from build123d import *

# Parameters (mm, degrees)
SKETCH_1_R               = 1.55
SKETCH_1_R_2             = 1.1
EXTRUDE_1_DEPTH          = 3
EXTRUDE_START            = 4.5
SKETCH_2_R               = 6
EXTRUDE_2_DEPTH          = 4.5
SKETCH_3_R               = 5.5
EXTRUDE_3_DEPTH          = 2.5
SKETCH_5_R               = 0.4
CUT_EXTRUDE_1_DEPTH      = 5
PATTERN_CIRCULAR_2_COUNT = 25
SKETCH_4_R               = 2.6
CUT_EXTRUDE_2_DEPTH      = 5
CUT_EXTRUDE_START        = -30
SKETCH_6_R               = 1.55
CUT_EXTRUDE_3_DEPTH      = 30
SKETCH_7_R               = 0.925
CUT_EXTRUDE_4_DEPTH      = 6
SKETCH_8_W               = 1.6
SKETCH_8_H               = 4.2
CUT_EXTRUDE_5_DEPTH      = 3.2
SKETCH_9_W               = 1.6
SKETCH_9_H               = 4.2
CUT_EXTRUDE_6_DEPTH      = 3.2


with BuildPart() as part:
    # 草图1 → 凸台-拉伸1 (new body)
    with BuildSketch(Plane.XY):
        with BuildLine():
            Line((4.472135955, 4), (19, 4))
            ThreePointArc((19, 4), (23, 0), (19, -4))
            Line((19, -4), (4.472135955, -4))
            ThreePointArc((4.472135955, -4), (0, -6), (-4.472135955, -4))
            Line((-4.472135955, -4), (-19, -4))
            ThreePointArc((-19, -4), (-23, 0), (-19, 4))
            Line((-19, 4), (-4.472135955, 4))
            ThreePointArc((-4.472135955, 4), (0, 6), (4.472135955, 4))
        make_face()
        Circle(SKETCH_1_R, mode=Mode.SUBTRACT)
        with Locations((19, 0)):
            Circle(SKETCH_1_R_2, mode=Mode.SUBTRACT)
        with Locations((-19, 0)):
            Circle(SKETCH_1_R_2, mode=Mode.SUBTRACT)
    extrude(amount=EXTRUDE_1_DEPTH)

    # 草图2 → 凸台-拉伸2 (add)
    with BuildSketch(Plane(origin=(0, 0, 0), x_dir=(-1, 0, 0), z_dir=(0, 0, -1)).offset(EXTRUDE_START)):
        Circle(SKETCH_2_R)
    extrude(amount=-EXTRUDE_2_DEPTH)

    # 草图3 → 凸台-拉伸3 (add)
    with BuildSketch(Plane(origin=(0, 0, -4.5), x_dir=(-1, 0, 0), z_dir=(0, 0, -1))):
        Circle(SKETCH_3_R)
    extrude(amount=EXTRUDE_3_DEPTH)

    # 草图5 → 切除-拉伸1 (cut)
    with BuildSketch(Plane(origin=(0, 0, -7), x_dir=(-1, 0, 0), z_dir=(0, 0, -1))):
        with Locations((0, 2.6)):
            Circle(SKETCH_5_R)
    cut_extrude_1 = extrude(amount=-CUT_EXTRUDE_1_DEPTH, mode=Mode.SUBTRACT)

    # 阵列(圆周)2: 切除-拉伸1 ×25 about axis
    pattern_circular_2_axis = Axis((0, 0, 0), (0, 0, 1))
    for i in range(1, PATTERN_CIRCULAR_2_COUNT):
        add(cut_extrude_1.rotate(pattern_circular_2_axis, i * 360 / PATTERN_CIRCULAR_2_COUNT), mode=Mode.SUBTRACT)

    # 草图4 → 切除-拉伸2 (cut)
    with BuildSketch(Plane(origin=(0, 0, -7), x_dir=(-1, 0, 0), z_dir=(0, 0, -1))):
        Circle(SKETCH_4_R)
    extrude(amount=-CUT_EXTRUDE_2_DEPTH, mode=Mode.SUBTRACT)

    # 草图6 → 切除-拉伸3 (cut)
    with BuildSketch(Plane.XY.offset(3).offset(CUT_EXTRUDE_START)):
        with Locations(Location((0, 0, 0), (0, 0, 180))):
            Circle(SKETCH_6_R)
    extrude(amount=CUT_EXTRUDE_3_DEPTH, mode=Mode.SUBTRACT)

    # 草图7 → 切除-拉伸4 (cut)
    with BuildSketch(Plane.XY.offset(3)):
        with Locations((5, 0)):
            Circle(SKETCH_7_R)
        with Locations((-5, 0)):
            Circle(SKETCH_7_R)
    extrude(amount=-CUT_EXTRUDE_4_DEPTH, mode=Mode.SUBTRACT)

    # 草图8 → 切除-拉伸5 (cut)
    with BuildSketch(Plane(origin=(6, 0, 0), x_dir=(0, 0, -1), z_dir=(1, 0, 0))):
        with Locations((0.8, 0)):
            Rectangle(SKETCH_8_W, SKETCH_8_H)
    extrude(amount=-CUT_EXTRUDE_5_DEPTH, mode=Mode.SUBTRACT)

    # 草图9 → 切除-拉伸6 (cut)
    with BuildSketch(Plane.ZY.offset(6)):
        with Locations((-0.8, 0)):
            Rectangle(SKETCH_9_W, SKETCH_9_H)
    extrude(amount=-CUT_EXTRUDE_6_DEPTH, mode=Mode.SUBTRACT)


solid = part.part
Can you work these out from the model? Positions are in its coordinate system, mm. A direction names the side the tool comes from. Give positions to 0.01 mm unless a question says otherwise; leave off trailing zeros. Order: outer loops, then holes, each group sorted by start corner. A loop starts at its lowest first (then second) coordinate and runs counter-clockwise, first axis right, second up. Notation, with made-up numbers: M 36,-15.5 L 53,-15.5 A23 ccw 53,-4.5 Z; hole C 30,-30 d10. An arc over 180 degrees is marked long. Use one line per item in the form item = value. Start each with the question number.
Item 1: If we section it at D-D (x = 7): Write out the boundary of the cut face in (y, z).
Item 2: For faces 1 (the flat face through (-3, -5, -4.5)), 2 (the flat face through (-5, 0, -3)), 3 (the flat face through (12, 4, 1)), which set-ups out of +Z, -Z, +X, -X, +Y, -Y let a thin tool reach every point of the face, with its end or its side?
Item 3: If I drill on line 1 along X through (y, z) = (0, -0.65); line 2 along Y through (x, z) = (0, -0.75); line 3 along Z through (x, y) = (7.5, -0.75), over which ranges is the centre line in solid material (lowest first)?
Item 4: If we section it at B-B (z = -3.5): Write out the boundary of the cut face in (x, y), then the cut area to 3 significant figures.
Item 5: If we section it at A-A (x = 19.5): Write out the boundary of the cut face in (y, z).
Item 6: If we section it at C-C (y = -3.5): Write out the boundary of the cut face in (x, z), then the cut area to 3 significant figures.
Item 7: Will these pins go through, and if not, where does the flat tip stop? pin 1 Ø2 at (x, y) = (-8, -1) entering from -Z; pin 2 Ø2 at (x, z) = (-18, 1) entering from -Y; pin 3 Ø1.7 at (x, y) = (-5, 0) entering from +Z; pin 4 Ø1.3 at (x, y) = (19, 0) entering from +Z.
Item 8: We'd pull the mould along X, two halves only. Please class faces 4 (the flat face through (-2.8, 0, -1)), 5 (the flat face through (12, -4, 1)), 6 (the flat face through (5, 0, -3)): +X half, -X half, draft (parallel to the pull), parting line (faces both ways), or undercut.
Outcome:
q1.outline = M -4,0 L 4,0 L 4,3 L -4,3 Z
q2.face_1 = -Z
q2.face_2 = +Z
q2.face_3 = +Z, -Z, +X, +Y
q3.line_1 = -2.8 to -1.55, 1.55 to 2.8
q3.line_2 = -6 to -1.55, 1.55 to 6
q3.line_3 = 0 to 3
q4.outline = C 0,0 d12; hole M -2.81,-0.18 A0.4 ccw -2.67,-0.87 A0.4 ccw -2.37,-1.51 A0.4 ccw -1.92,-2.05 A0.4 ccw -1.35,-2.46 A0.4 ccw -0.7,-2.72 A0.4 ccw 0,-2.81 A0.4 ccw 0.7,-2.72 A0.4 ccw 1.35,-2.46 A0.4 ccw 1.92,-2.05 A0.4 ccw 2.37,-1.51 A0.4 ccw 2.67,-0.87 A0.4 ccw 2.81,-0.18 A0.4 ccw 2.76,0.53 A0.4 ccw 2.54,1.2 A0.4 ccw 2.17,1.79 A0.4 ccw 1.65,2.27 A0.4 ccw 1.03,2.61 A0.4 ccw 0.35,2.79 A0.4 ccw -0.35,2.79 A0.4 ccw -1.03,2.61 A0.4 ccw -1.65,2.27 A0.4 ccw -2.17,1.79 A0.4 ccw -2.54,1.2 A0.4 ccw -2.76,0.53 A0.4 ccw Z
q4.area = 85.9 mm2
q5.outline = M -3.97,0 L -0.98,0 L -0.98,3 L -3.97,3 Z; M 0.98,0 L 3.97,0 L 3.97,3 L 0.98,3 Z
q6.outline = M -20.94,0 L -4.87,0 L -4.87,-4.5 L -4.24,-4.5 L -4.24,-7 L 4.24,-7 L 4.24,-4.5 L 4.87,-4.5 L 4.87,0 L 20.94,0 L 20.94,3 L -20.94,3 Z
q6.area = 191 mm2
q7.pin_1 = 0
q7.pin_2 = -4
q7.pin_3 = -3
q7.pin_4 = through
q8.face_4 = -X half
q8.face_5 = draft
q8.face_6 = undercut
